```python
from build123d import *

# Parameters (mm, degrees)
SALIENTE_EXTRUIR1_DEPTH = 200
CROQUIS2_W              = 178
CROQUIS2_H              = 120
SALIENTE_EXTRUIR2_DEPTH = 11
CROQUIS3_W              = 170
CROQUIS3_H              = 115
CORTAR_EXTRUIR1_DEPTH   = 9
CROQUIS4_W              = 2.5
CROQUIS4_H              = 170
CROQUIS4_H_2            = 180
CORTAR_EXTRUIR2_DEPTH   = 42.5
CROQUIS5_R              = 3.075
CORTAR_EXTRUIR3_DEPTH   = 10
CORTAR_EXTRUIR4_DEPTH   = 11.2
CROQUIS7_R              = 2.55
CORTAR_EXTRUIR5_DEPTH   = 10
CROQUIS9_W              = 107
CROQUIS9_H              = 16
CORTAR_EXTRUIR7_DEPTH   = 4
CROQUIS8_R              = 3
CROQUIS8_R_2            = 2.5
CROQUIS8_R_3            = 3.4
CORTAR_EXTRUIR6_DEPTH   = 4
CROQUIS11_OUTSIDE_W     = 256.562
CROQUIS11_OUTSIDE_H     = 236.562
CORTAR_EXTRUIR10_DEPTH  = 1
CORTAR_EXTRUIR11_DEPTH  = 0.5
CROQUIS13_W             = 21.552052497
CROQUIS13_H             = 68.530716877
CROQUIS13_W_2           = 18.933824997
CROQUIS13_H_2           = 79.190643128
CORTAR_EXTRUIR12_DEPTH  = 201
CROQUIS18_R             = 1.75
CORTAR_EXTRUIR13_DEPTH  = 3.5
CROQUIS21_W             = 95.6
CROQUIS21_H             = 8.5
SALIENTE_EXTRUIR3_DEPTH = 5
CROQUIS22_W             = 79.935638501
CROQUIS22_H             = 8.5
SALIENTE_EXTRUIR4_DEPTH = 8
SALIENTE_EXTRUIR5_DEPTH = 107
CROQUIS25_R             = 3
SALIENTE_EXTRUIR6_DEPTH = 1.5
MATRIZL1_COUNT          = 8
MATRIZL1_PITCH          = 12
CHAFL_N1_SIZE           = 1


with BuildPart() as part:
    # Croquis1 → Saliente-Extruir1 (new body)
    with BuildSketch(Plane(origin=(0, 0, 0), x_dir=(0, 0, -1), z_dir=(1, 0, 0))):
        Polygon((-90, 6.926136028), (-90, 45), (90, 45), (90, 6.926136028), (87.7, 5), (87.7, 0), (85.2, 0), (85.2, 6.167243447), (87.5, 8.093379476), (87.5, 42.5), (-87.5, 42.5), (-87.5, 8.093379476), (-85.2, 6.167243447), (-85.2, 0), (-87.7, 0), (-87.7, 5), align=None)
    extrude(amount=SALIENTE_EXTRUIR1_DEPTH)

    # Croquis2 → Saliente-Extruir2 (add)
    with BuildSketch(Plane(origin=(0, 45, 0), x_dir=(1, 0, 0), z_dir=(0, 1, 0))):
        with Locations((100, 0)):
            Rectangle(CROQUIS2_W, CROQUIS2_H)
    extrude(amount=-SALIENTE_EXTRUIR2_DEPTH)

    # Croquis3 → Cortar-Extruir1 (cut)
    with BuildSketch(Plane(origin=(0, 45, 0), x_dir=(1, 0, 0), z_dir=(0, 1, 0))):
        with Locations((100, 0)):
            Rectangle(CROQUIS3_W, CROQUIS3_H)
    extrude(amount=-CORTAR_EXTRUIR1_DEPTH, mode=Mode.SUBTRACT)

    # Croquis4 → Cortar-Extruir2 (cut)
    with BuildSketch(Plane(origin=(0, 0, 0), x_dir=(-1, 0, 0), z_dir=(0, -1, 0))):
        with Locations((-198.75, -5)):
            Rectangle(CROQUIS4_W, CROQUIS4_H)
        with Locations((-1.25, 0)):
            Rectangle(CROQUIS4_W, CROQUIS4_H_2)
    extrude(amount=-CORTAR_EXTRUIR2_DEPTH, mode=Mode.SUBTRACT)

    # Croquis5 → Cortar-Extruir3 (cut)
    with BuildSketch(Plane(origin=(0, 45, 0), x_dir=(1, 0, 0), z_dir=(0, 1, 0))):
        with Locations((181.925, 78.75)):
            Circle(CROQUIS5_R)
        with Locations((169.925, 78.75)):
            Circle(CROQUIS5_R)
        with Locations((157.925, 78.75)):
            Circle(CROQUIS5_R)
        with Locations((145.925, 78.75)):
            Circle(CROQUIS5_R)
        with Locations((133.925, 78.75)):
            Circle(CROQUIS5_R)
        with Locations((121.925, 78.75)):
            Circle(CROQUIS5_R)
        with Locations((109.925, 78.75)):
            Circle(CROQUIS5_R)
        with Locations((97.925, 78.75)):
            Circle(CROQUIS5_R)
    extrude(amount=-CORTAR_EXTRUIR3_DEPTH, mode=Mode.SUBTRACT)

    # Croquis6 → Cortar-Extruir4 (cut)
    with BuildSketch(Plane.XZ.offset(-34)):
        Polygon((185.925, -81.059401077), (185.925, -76.440598923), (181.925, -74.131197846), (177.925, -76.440598923), (177.925, -81.059401077), (181.925, -83.368802154), align=None)
        Polygon((169.925, -74.131197846), (165.925, -76.440598923), (165.925, -81.059401077), (169.925, -83.368802154), (173.925, -81.059401077), (173.925, -76.440598923), align=None)
        Polygon((157.925, -74.131197846), (153.925, -76.440598923), (153.925, -81.059401077), (157.925, -83.368802154), (161.925, -81.059401077), (161.925, -76.440598923), align=None)
        Polygon((145.925, -74.131197846), (141.925, -76.440598923), (141.925, -81.059401077), (145.925, -83.368802154), (149.925, -81.059401077), (149.925, -76.440598923), align=None)
        Polygon((133.925, -74.131197846), (129.925, -76.440598923), (129.925, -81.059401077), (133.925, -83.368802154), (137.925, -81.059401077), (137.925, -76.440598923), align=None)
        Polygon((121.925, -74.131197846), (117.925, -76.440598923), (117.925, -81.059401077), (121.925, -83.368802154), (125.925, -81.059401077), (125.925, -76.440598923), align=None)
        Polygon((109.925, -74.131197846), (105.925, -76.440598923), (105.925, -81.059401077), (109.925, -83.368802154), (113.925, -81.059401077), (113.925, -76.440598923), align=None)
        Polygon((97.925, -74.131197846), (93.925, -76.440598923), (93.925, -81.059401077), (97.925, -83.368802154), (101.925, -81.059401077), (101.925, -76.440598923), align=None)
    extrude(amount=-CORTAR_EXTRUIR4_DEPTH, mode=Mode.SUBTRACT)

    # Croquis7 → Cortar-Extruir5 (cut)
    with BuildSketch(Plane(origin=(0, 45, 0), x_dir=(1, 0, 0), z_dir=(0, 1, 0))):
        with Locations((82.885064516, 78.75)):
            Circle(CROQUIS7_R)
        with Locations((73.551483871, 78.75)):
            Circle(CROQUIS7_R)
        with Locations((64.217903226, 78.75)):
            Circle(CROQUIS7_R)
        with Locations((54.88432258, 78.75)):
            Circle(CROQUIS7_R)
        with Locations((45.550741935, 78.75)):
            Circle(CROQUIS7_R)
        with Locations((36.21716129, 78.75)):
            Circle(CROQUIS7_R)
        with Locations((26.883580645, 78.75)):
            Circle(CROQUIS7_R)
        with Locations((17.55, 78.75)):
            Circle(CROQUIS7_R)
    extrude(amount=-CORTAR_EXTRUIR5_DEPTH, mode=Mode.SUBTRACT)

    # Croquis9 → Cortar-Extruir7 (cut)
    with BuildSketch(Plane(origin=(0, 45, 0), x_dir=(1, 0, 0), z_dir=(0, 1, 0))):
        with Locations((131.5, -73)):
            Rectangle(CROQUIS9_W, CROQUIS9_H)
    extrude(amount=-CORTAR_EXTRUIR7_DEPTH, mode=Mode.SUBTRACT)

    # Croquis8 → Cortar-Extruir6 (cut)
    with BuildSketch(Plane(origin=(0, 45, 0), x_dir=(1, 0, 0), z_dir=(0, 1, 0))):
        with Locations((60, -73)):
            Circle(CROQUIS8_R)
        with Locations((37.5, -73)):
            Circle(CROQUIS8_R_2)
        with Locations((23.1, -73)):
            Circle(CROQUIS8_R_3)
        with Locations((47.5, -73)):
            Circle(CROQUIS8_R)
        with Locations((70, -78.5)):
            Circle(CROQUIS8_R_2)
        with Locations((70, -67.5)):
            Circle(CROQUIS8_R_2)
    extrude(amount=-CORTAR_EXTRUIR6_DEPTH, mode=Mode.SUBTRACT)

    # Croquis11 outside → Cortar-Extruir10 (cut)
    with BuildSketch(Plane.XZ.offset(-42.5)):
        with Locations((100, 0)):
            Rectangle(CROQUIS11_OUTSIDE_W, CROQUIS11_OUTSIDE_H)
        Polygon((47.5, 4691.358777844), (-3952.116025404, 2382.179388922), (-3952.116025404, -2236.179388922), (47.5, -4545.358777844), (4047.116025404, -2236.179388922), (4047.116025404, 2382.179388922), align=None, mode=Mode.SUBTRACT)
        Polygon((47.5, 68.381197846), (51.5, 70.690598923), (51.5, 75.309401077), (47.5, 77.618802154), (43.5, 75.309401077), (43.5, 70.690598923), align=None)
    extrude(amount=-CORTAR_EXTRUIR10_DEPTH, mode=Mode.SUBTRACT)

    # Croquis12 → Cortar-Extruir11 (cut)
    with BuildSketch(Plane(origin=(0, 45, 0), x_dir=(1, 0, 0), z_dir=(0, 1, 0))):
        with BuildLine():
            Line((68.102067459, -82.021058373), (58.056221043, -76.606112981))
            ThreePointArc((58.056221043, -76.606112981), (55.903376089, -73), (58.056221043, -69.393887019))
            Line((58.056221043, -69.393887019), (68.102067459, -63.978941627))
            ThreePointArc((68.102067459, -63.978941627), (72.050398722, -64.065489106), (74, -67.5))
            Line((74, -67.5), (74, -78.5))
            ThreePointArc((74, -78.5), (72.050398722, -81.934510894), (68.102067459, -82.021058373))
        make_face()
        with BuildLine():
            Line((47.5, -77), (37.5, -77))
            ThreePointArc((37.5, -77), (33.5, -73), (37.5, -69))
            Line((37.5, -69), (47.5, -69))
            ThreePointArc((47.5, -69), (51.5, -73), (47.5, -77))
        make_face()
    extrude(amount=-CORTAR_EXTRUIR11_DEPTH, mode=Mode.SUBTRACT)

    # Croquis13 → Cortar-Extruir12 (cut, through all)
    with BuildSketch(Plane.ZY):
        with Locations((-79.223973752, 8.234641561)):
            Rectangle(CROQUIS13_W, CROQUIS13_H)
        with Locations((80.533087502, 2.904678436)):
            Rectangle(CROQUIS13_W_2, CROQUIS13_H_2)
    extrude(amount=-CORTAR_EXTRUIR12_DEPTH, mode=Mode.SUBTRACT)

    # Croquis18 → Cortar-Extruir13 (cut, through all)
    with BuildSketch(Plane.XZ.offset(-42.5)):
        with Locations((191.36, -82)):
            Circle(CROQUIS18_R)
        with Locations((8.64, -82)):
            Circle(CROQUIS18_R)
        with Locations((8.64, 82)):
            Circle(CROQUIS18_R)
        with Locations((191.36, 82)):
            Circle(CROQUIS18_R)
    extrude(amount=-CORTAR_EXTRUIR13_DEPTH, mode=Mode.SUBTRACT)

    # Croquis21 → Saliente-Extruir3 (add)
    with BuildSketch(Plane(origin=(0, 0, -60), x_dir=(-1, 0, 0), z_dir=(0, 0, -1))):
        with Locations((-58.8, 38.25)):
            Rectangle(CROQUIS21_W, CROQUIS21_H)
    extrude(amount=SALIENTE_EXTRUIR3_DEPTH)

    # Croquis22 → Saliente-Extruir4 (add)
    with BuildSketch(Plane.ZY.offset(-11)):
        with Locations((-25.03218075, 38.25)):
            Rectangle(CROQUIS22_W, CROQUIS22_H)
    extrude(amount=SALIENTE_EXTRUIR4_DEPTH)

    # Croquis24 → Saliente-Extruir5 (add)
    with BuildSketch(Plane(origin=(78, 0, 0), x_dir=(0, 0, -1), z_dir=(1, 0, 0))):
        Polygon((-84.5, 42.5), (-83, 41), (-76, 41), (-76, 44), (-80, 44), (-81, 45), (-81, 42.5), align=None)
    extrude(amount=SALIENTE_EXTRUIR5_DEPTH)

    # Croquis25 → Saliente-Extruir6 (add)
    with BuildSketch(Plane(origin=(0, 45, 0), x_dir=(1, 0, 0), z_dir=(0, 1, 0))):
        Polygon((181.925, 74.131197846), (185.925, 76.440598923), (185.925, 81.059401077), (181.925, 83.368802154), (177.925, 81.059401077), (177.925, 76.440598923), align=None)
        with Locations((181.925, 78.75)):
            Circle(CROQUIS25_R, mode=Mode.SUBTRACT)
    saliente_extruir6 = extrude(amount=-SALIENTE_EXTRUIR6_DEPTH)

    # MatrizL1: Saliente-Extruir6 ×8
    with Locations(*[(-i * MATRIZL1_PITCH, 0, 0) for i in range(1, MATRIZL1_COUNT)]):
        add(saliente_extruir6)

    # Chaflán1
    chafl_n1_edges = [part.edges().sort_by_distance(p)[0] for p in [
        (0, 43.75, 90),
        (0, 45, 0),
        (0, 43.75, -90),
        (100, 45, 90),
        (100, 45, -90),
        (200, 43.75, -90),
        (200, 45, 0),
        (200, 43.75, 90),
    ]]
    chamfer(chafl_n1_edges, length=CHAFL_N1_SIZE)


solid = part.part
```
Work out the finished part from the listing and answer in its coordinate system (mm). A direction names the side the tool comes from. Coordinates: 2 decimals unless noted, no trailing zeros. Write each loop counter-clockwise with the first axis right and the second up, starting at its lowest first coordinate (ties: lowest second). Pieces come first, ordered by that corner, then holes.
Q1. Determine the mould class of faces 1 (the face through (147, 38, -60)), 2 (the face through (15.002, 43.768, -78.862)) for opening direction Z: released by +Z, released by -Z, zero draft, split by the parting line, or undercut.
Q2. A cutting plane is placed at B-B, the plane z = 4.5. Give the vertices of the cut face in (x, y).
Q3. Each of these flat-tipped pins is pushed along its axis until it touches: pin 1 Ø1.2 at (x, z) = (155, 77.5) entering from +Y; pin 2 Ø6 at (x, z) = (77.5, -39) entering from +Y; pin 3 Ø1.5 at (x, y) = (100, 35.5) entering from -Z. Where does it stop, or does it pass through?
Q4. Find the intervals of material crossed by line 1 (Z direction, x = 41, y = 36.5); line 2 (X direction, y = 43.5, z = 78.5); line 3 (X direction, y = 41.25, z = -23), in increasing order.
Q5. A cutting plane is placed at A-A, the plane y = 38.5. Give the vertices of the cut face in (x, z).
Q6. Which of the six approach directions +Z, -Z, +X, -X, +Y, -Y give full straight-line access (tool end or side, diameter ignored) to faces 3 (the face through (43, 44.5, 73)), 4 (the face through (99, 38, 60)), 5 (the face through (46.56, 43.5, 69.99))?
Findings below:
1. face 1: released by -Z
1. face 2: undercut
2. outline: (0, 42.5) - (3, 42.5) - (3, 34) - (189, 34) - (189, 42.5) - (200, 42.5) - (200, 44) - (199, 45) - (185, 45) - (185, 36) - (15, 36) - (15, 45) - (1, 45) - (0, 44) - close
3. pin 1: stops at y = 44
3. pin 2: stops at y = 36
3. pin 3: stops at z = -65
4. line 1: z = -65 to -57.5, 57.5 to 60
4. line 2: x = 0 to 67.5, 72.5 to 200
4. line 3: x = 3 to 15, 185 to 189
5. outline: (3, -65) - (106.6, -65) - (106.6, -60) - (189, -60) - (189, 60) - (11, 60) - (11, 14.94) - (3, 14.94) - close; hole (15, -57.5) - (185, -57.5) - (185, 57.5) - (15, 57.5) - close
6. face 3: +Y
6. face 4: +X, -X, -Y
6. face 5: -Y
